Build history of the part. All positions in model axes, mm. Coordinates: 2 decimals unless noted, no trailing zeros. Loops run counter-clockwise (first coordinate to the right, second up) from the corner with the lowest first, then second, coordinate; pieces in that order, holes last.
(1) Wall check: L1, parallel to X at y = -0.45, z = 224.5; L2, parallel to Z at x = -94, y = 0.5 (3 decimals); L3, parallel to Z at x = 5.5, y = 0.4 (3 decimals). Give the ranges that are in metal, low to high.
(2) Slice it at A-A (y = -0.6). Give the cut face in (x, z) (1 decimal), and give its area (3 significant figures).
(3) Flat gauge pins, fed straight in: P1, Ø1, axis at y = 0.5, z = 218, coming from the -X side; P2, Ø1.6, axis at y = 0, z = 191, coming from the +X side; P3, Ø1.5, axis at x = 7, y = 1, coming from the -Z side (3 decimals). Where does each tip first touch, or does it go through?
(4) Slice it at B-B (x = -112). Give the cut face in (y, z) (1 decimal), and give its area (3 significant figures).
from build123d import *

# Parameters (mm, degrees)
SKETCH1_W           = 315.575
SKETCH1_H           = 3.175
BOSS_EXTRUDE1_DEPTH = 235.775
SKETCH3_W           = 25.4
SKETCH3_H           = 3.175
SKETCH3_W_2         = 61.575
CUT_EXTRUDE1_DEPTH  = 3.175
CUT_EXTRUDE2_START  = -3.175
SKETCH5_W           = 2.286
SKETCH5_H           = 118.364
CUT_EXTRUDE2_DEPTH  = 287.894626403
SKETCH6_W           = 48.454093678
SKETCH6_H           = 25
CUT_EXTRUDE4_DEPTH  = 284.719626403


with BuildPart() as part:
    # Sketch1 → Boss-Extrude1 (new body)
    with BuildSketch(Plane.XY):
        Rectangle(SKETCH1_W, SKETCH1_H)
    extrude(amount=BOSS_EXTRUDE1_DEPTH)

    # Sketch3 → Cut-Extrude1 (cut)
    with BuildSketch(Plane(origin=(0, 0, 0), x_dir=(-1, 0, 0), z_dir=(0, 0, -1))):
        with Locations((-145.0875, 0)):
            Rectangle(SKETCH3_W, SKETCH3_H)
        Rectangle(SKETCH3_W_2, SKETCH3_H)
        with Locations((145.0875, 0)):
            Rectangle(SKETCH3_W, SKETCH3_H)
    extrude(amount=-CUT_EXTRUDE1_DEPTH, mode=Mode.SUBTRACT)

    # Sketch5 → Cut-Extrude2 (cut)
    with BuildSketch(Plane(origin=(0, 1.5875, 0), x_dir=(1, 0, 0), z_dir=(0, 1, 0)).offset(CUT_EXTRUDE2_START)):
        with Locations((-156.6445, -176.593)):
            Rectangle(SKETCH5_W, SKETCH5_H)
    cut_extrude2 = extrude(amount=CUT_EXTRUDE2_DEPTH, mode=Mode.SUBTRACT)

    # Mirror1: Cut-Extrude2 across plane
    add(cut_extrude2.mirror(Plane(origin=(0, 0, 0), x_dir=(0, 0, 1), z_dir=(1, 0, 0))), mode=Mode.SUBTRACT)

    # Sketch6 → Cut-Extrude4 (cut, through all)
    with BuildSketch(Plane(origin=(0, 1.5875, 0), x_dir=(1, 0, 0), z_dir=(0, 1, 0))):
        with Locations((-97.616032964, -223.275)):
            Rectangle(SKETCH6_W, SKETCH6_H)
    cut_extrude4 = extrude(amount=-CUT_EXTRUDE4_DEPTH, mode=Mode.SUBTRACT)

    # Mirror2: Cut-Extrude4 across plane
    add(cut_extrude4.mirror(Plane(origin=(0, 0, 0), x_dir=(0, 0, 1), z_dir=(1, 0, 0))), mode=Mode.SUBTRACT)


solid = part.part
Response values:
1. L1: x = -155.5 to -121.84, -73.39 to 73.39, 121.84 to 155.5
1. L2: z = 0 to 210.775
1. L3: z = 3.175 to 235.775
2. outline: (-157.8, 3.2) - (-132.4, 3.2) - (-132.4, 0) - (-30.8, 0) - (-30.8, 3.2) - (30.8, 3.2) - (30.8, 0) - (132.4, 0) - (132.4, 3.2) - (157.8, 3.2) - (157.8, 117.4) - (155.5, 117.4) - (155.5, 235.8) - (121.8, 235.8) - (121.8, 210.8) - (73.4, 210.8) - (73.4, 235.8) - (-73.4, 235.8) - (-73.4, 210.8) - (-121.8, 210.8) - (-121.8, 235.8) - (-155.5, 235.8) - (-155.5, 117.4) - (-157.8, 117.4) - close
2. area: 71,100 mm2
3. P1: stops at x = -155.5
3. P2: stops at x = 155.5
3. P3: stops at z = 3.175
4. outline: (-1.6, 0) - (1.6, 0) - (1.6, 210.8) - (-1.6, 210.8) - close
4. area: 669 mm2
